```python
from build123d import *

# Parameters (mm, degrees)
F0_W         = 101.6
F0_H         = 101.6
F0_R         = 21.59
F1_DEPTH     = 2.54
F3_R         = 3.175
F4_DEPTH     = 31.75
F5_R         = 2.54
F6_T1_DEPTH  = 123.5970452561
F6_T3_DEPTH  = 85.4970452561
F6_T5_DEPTH  = 85.4970452561
F6_T10_DEPTH = 123.5970452561
F6_S11_R     = 3.175
F6_T12_DEPTH = 63
F8_D         = 2.794


# Not quite as in the source:
# - a fillet or chamfer that OpenCascade refuses, or shapes differently, is made with other operations: its cross-section is extruded or revolved along the edge and cut away or added


with BuildPart() as f1:
    # F0 (on Top) → F1 (new body)
    with BuildSketch(Plane.XY):
        Rectangle(F0_W, F0_H)
        with Locations((0, -12.7)):
            Circle(F0_R, mode=Mode.SUBTRACT)
        Polygon((-50.8, 50.8), (50.8, 50.8), (0, 88.9), align=None)
    extrude(amount=F1_DEPTH)

    # F2: fillet of radius 4.826 on 1 edges, made by hand

    # F2_s1 → F2_t2 (revolve, cut)
    with BuildSketch(Plane.XZ.offset(12.7)):
        with BuildLine():
            ThreePointArc((21.59, 0), (23.3645471712, 1.8566146333), (25.8402329348, 2.54))
            Line((25.8402329348, 2.54), (21.59, 2.54))
            Line((21.59, 2.54), (21.59, 0))
        make_face()
    revolve(axis=Axis((0, -12.7, 2.54), (0, 0, 1)), mode=Mode.SUBTRACT)

    # F3 (on face) → F4 (join)
    with BuildSketch(Plane.XY.offset(2.54)):
        with Locations((0, -43.2976202148)):
            Circle(F3_R)
    extrude(amount=F4_DEPTH)

    # F5
    f5_edges = [f1.edges().sort_by_distance(p)[0] for p in [
        (-3.175, -43.29762, 34.29),
    ]]
    fillet(f5_edges, radius=F5_R)

    # F6: fillet of radius 5.08 on 5 edges, made by hand

    # F6_s2 → F6_t1 (cut)
    with BuildSketch(Plane.XZ.offset(-61.7985226281)):
        with BuildLine():
            ThreePointArc((46.4005909488, 2.54), (48.9405909488, 1.8594090512), (50.8, 0))
            Line((50.8, 0), (50.8, 2.54))
            Line((50.8, 2.54), (46.4005909488, 2.54))
        make_face()
        with BuildLine():
            ThreePointArc((-46.4005909488, 2.54), (-48.9405909488, 1.8594090512), (-50.8, 0))
            Line((-50.8, 0), (-50.8, 2.54))
            Line((-50.8, 2.54), (-46.4005909488, 2.54))
        make_face()
    extrude(amount=F6_T1_DEPTH, mode=Mode.SUBTRACT)

    # F6_s4 → F6_t3 (cut)
    with BuildSketch(Plane(origin=(51.4708181025, 38.6031135768, 0), x_dir=(0, 0, 1), z_dir=(-0.8, -0.6, 0))):
        with BuildLine():
            ThreePointArc((2.54, 66.7205909488), (1.8594090512, 69.2605909488), (0, 71.12))
            Line((0, 71.12), (2.54, 71.12))
            Line((2.54, 71.12), (2.54, 66.7205909488))
        make_face()
    extrude(amount=F6_T3_DEPTH, mode=Mode.SUBTRACT)

    # F6_s6 → F6_t5 (cut)
    with BuildSketch(Plane(origin=(16.9268181025, -12.6951135768, 0), x_dir=(0, 0, 1), z_dir=(-0.8, 0.6, 0))):
        with BuildLine():
            ThreePointArc((2.54, 66.7205909488), (1.8594090512, 69.2605909488), (0, 71.12))
            Line((0, 71.12), (2.54, 71.12))
            Line((2.54, 71.12), (2.54, 66.7205909488))
        make_face()
    extrude(amount=F6_T5_DEPTH, mode=Mode.SUBTRACT)


with BuildPart() as f6_tool8:
    # F6_s9 → F6_t10 (new body)
    with BuildSketch(Plane.YZ.offset(-61.7985226281)):
        with BuildLine():
            ThreePointArc((-46.4005909488, 2.54), (-48.9405909488, 1.8594090512), (-50.8, 0))
            Line((-50.8, 0), (-50.8, 2.54))
            Line((-50.8, 2.54), (-46.4005909488, 2.54))
        make_face()
    extrude(amount=F6_T10_DEPTH)

    # F6_s11 → F6_t12 (cut, symmetric)
    with BuildSketch(Plane.XY.offset(1.3)):
        with Locations((0, -43.2976202148)):
            Circle(F6_S11_R)
    extrude(amount=F6_T12_DEPTH, both=True, mode=Mode.SUBTRACT)


with BuildPart() as f1_1:
    add(f1.part)

    # F6_t7: cut F6_tool8
    add(f6_tool8.part, mode=Mode.SUBTRACT)

    # F8 (through all)
    with Locations(Plane(origin=(0, 0, 0), x_dir=(1, 0, 0), z_dir=(0, 0, -1))):
        with Locations((-49.53, -45.4025), (-49.53, 0), (-49.53, 45.72), (49.53, 45.72), (49.53, 0), (49.53, -45.4025)):
            Hole(F8_D / 2)


solid = f1_1.part
```
Can you work these out from the model? Positions are in its coordinate system, mm. A direction names the side the tool comes from. Give positions to 0.01 mm unless a question says otherwise; leave off trailing zeros. Loops run counter-clockwise (first coordinate to the right, second up) from the corner with the lowest first, then second, coordinate; pieces in that order, holes last. Notation, with made-up numbers: M 57.25,13 L 98.25,13 A11 cw 98.25,32 Z; hole C 9,76 d1. An arc over 180 degrees is marked long. Use CSV: the item, a comma, the result in double quotes. Start each with the question number.
1. Imagine slicing it at B-B, the plane z = 13.5. Write out the boundary of the cut face in (x, y) (3 decimals), plus the area to 3 significant figures.
2. If we mould it in two halves opening along Y, with no side actions, what happens to faces 3 (the face through (48.134, 0.053, 0.885)), 4 (the face through (-1, 20, 0)), 5 (the face through (24.62, 68.07, 1.88))? For each: released by +Y, released by -Y, zero draft, split by the parting line, or undercut.
3. If I drill on L1, parallel to Z at x = 9, y = 54.5; L2, parallel to Y at x = 49.53, z = 0.65; L3, parallel to Y at x = -49, z = 1, over which ranges is the centre line in solid material (lowest first)?
4. On a 3-axis mill with a long thin cutter (end or side, diameter ignored), from which of +Z, -Z, +X, -X, +Y, -Y can I reach the whole of each face in a straight line? I mean faces 1 (the face through (1.707, -40.62, 16.94)), 2 (the face through (-48.134, -0.053, 0.885)). Say none if no direction works.
5. For P1, Ø3.5, axis at x = -49.53, y = 0, coming from the +Z side, with a flat end and sliding along its axis, tell me the tip position at first contact or that it passes through.
6. Imagine slicing it at A-A, the plane y = 34.5. Write out the boundary of the cut face in (x, z).
Response values:
1,outline,"C 0,-43.298 d6.35"
1,area,"31.7 mm^2"
2,face 3,"undercut"
2,face 4,"zero draft"
2,face 5,"released by +Y"
3,L1,"0 to 2.54"
3,L2,"-50.35 to -47.12, -44.32 to -1.4, 1.4 to 44.01, 46.8 to 51.2"
3,L3,"-50.04 to -47.01, -44.43 to -1.29, 1.29 to 44.11, 46.7 to 51.21"
4,face 1,"+Z"
4,face 2,"+Z, -Z"
5,P1,"z = 2.35"
6,outline,"M -50.8,0 L 50.8,0 A5.08 ccw 46.4,2.54 L -46.4,2.54 A5.08 ccw Z"
